Geometry check sheet. Reference: the model listing, model coordinates, mm. Give positions to 0.01 mm unless a question says otherwise; leave off trailing zeros. Order: outer loops, then holes, each group sorted by start corner. A loop starts at its lowest first (then second) coordinate and runs counter-clockwise, first axis right, second up. Notation, with made-up numbers: M 55,76.25 L 97,76.25 A17 ccw 97,105.25 Z; hole C -27,57 d7. An arc over 180 degrees is marked long. Put each result on its own line as item: value. Start each with the question number.
Q1. Material ranges on L1, parallel to Y at x = 0, z = -3.9; L2, parallel to X at y = -0.5, z = -3.45; L3, parallel to X at y = 1.75, z = -1.6, recorded low to high.
Q2. Go/stop test with a flat-tipped pin: pin 1 (3 mm diameter, centred on x = -1.5, y = 1, fed in from -Z). Record where the tip stops, or that it passes through.
Q3. Section check A-A on z = -1.2. Record the cut outline in (x, y), then the cut area to 3 significant figures.
Q4. Mould release check, pull along Y, two halves, no side actions. Record for faces 1 (the flat face through (4.852, 2.854, -2.465)), 2 (the flat face through (3, 1, -5)), 3 (the cylindrical face through (-3, 0, -2)), 4 (the flat face through (4.898, -2.775, -2.465)): +Y half, -Y half, draft (parallel to the pull), parting line (faces both ways), or undercut.
Q5. Section check C-C on y = 4. Record the cut outline in (x, z).
Q6. Section check B-B on x = 0. Record the cut outline in (y, z), then the cut area to 3 significant figures.
```python
from build123d import *

# Parameters (mm, degrees)
F0_R     = 6.5
F1_DEPTH = 5
F3_DEPTH = 5.001
F4_R     = 3
F5_DEPTH = 5.001


with BuildPart() as f1:
    # F0 (on Top) → F1 (new body)
    with BuildSketch(Plane.XY):
        Circle(F0_R)
    extrude(amount=-F1_DEPTH)

    # F2 (on face) → F3 (cut, through all)
    with BuildSketch(Plane.XY):
        with BuildLine():
            Line((-3.25, 5.629165), (3.25, 5.629165))
            ThreePointArc((3.25, 5.629165), (0, 6.5), (-3.25, 5.629165))
        make_face()
        with BuildLine():
            Line((-6.5, 0), (-3.25, 5.629165))
            ThreePointArc((-3.25, 5.629165), (-5.629165, 3.25), (-6.5, 0))
        make_face()
        with BuildLine():
            ThreePointArc((-6.5, 0), (-5.629165, -3.25), (-3.25, -5.629165))
            Line((-3.25, -5.629165), (-6.5, 0))
        make_face()
        with BuildLine():
            ThreePointArc((-3.25, -5.629165), (0, -6.5), (3.25, -5.629165))
            Line((3.25, -5.629165), (-3.25, -5.629165))
        make_face()
        with BuildLine():
            ThreePointArc((3.25, -5.629165), (5.629165, -3.25), (6.5, 0))
            Line((6.5, 0), (3.25, -5.629165))
        make_face()
        with BuildLine():
            Line((3.25, 5.629165), (6.5, 0))
            ThreePointArc((6.5, 0), (5.629165, 3.25), (3.25, 5.629165))
        make_face()
    extrude(amount=-F3_DEPTH, mode=Mode.SUBTRACT)

    # F4 (on face) → F5 (cut, through all)
    with BuildSketch(Plane.XY):
        Circle(F4_R)
    extrude(amount=-F5_DEPTH, mode=Mode.SUBTRACT)


solid = f1.part
```
Results found:
1. L1: y = -5.63 to -3, 3 to 5.63
1. L2: x = -6.21 to -2.96, 2.96 to 6.21
1. L3: x = -5.49 to -2.44, 2.44 to 5.49
2. pin 1: stops at z = -5
3. outline: M -6.5,0 L -3.25,-5.63 L 3.25,-5.63 L 6.5,0 L 3.25,5.63 L -3.25,5.63 Z; hole C 0,0 d6
3. area: 81.5 mm^2
4. face 1: +Y half
4. face 2: draft
4. face 3: undercut
4. face 4: -Y half
5. outline: M -4.19,-5 L 4.19,-5 L 4.19,0 L -4.19,0 Z
6. outline: M -5.63,-5 L -3,-5 L -3,0 L -5.63,0 Z; M 3,-5 L 5.63,-5 L 5.63,0 L 3,0 Z
6. area: 26.3 mm^2
